Build history of the part. All positions in model axes, mm. Give positions to 0.01 mm unless a question says otherwise; leave off trailing zeros. Loops run counter-clockwise (first coordinate to the right, second up) from the corner with the lowest first, then second, coordinate; pieces in that order, holes last. Notation, with made-up numbers: (67.5, 65.25) - (75.5, 65.25) arc R24 cw to (75.5, 87.25) - close; hole circle Ø8 at (49.5, -27.5). An arc over 180 degrees is marked (long way). Return JSON: item names as keys, results as strings. Group by question number.
1) Slice it at A-A (x = -7). List the corners of the cut face in (y, z), and give its area (3 significant figures).
2) Slice it at B-B (y = -9.5). List the corners of the cut face in (x, z).
3) Drop a flat-ended pin along its axis: pin 1 (25 mm diameter, centred on x = -5.44, z = 0, fed in from -Y). Give the stop position or say it passes through.
4) Slice it at C-C (z = -1.5). List the corners of the cut face in (x, y), and give its area (3 significant figures).
5) Drill centre lines: probe 1 along Z at (x, y) = (-4.5, -39); probe 2 along Z at (x, y) = (7, -36); probe 3 along X at (y, z) = (-14.5, -2). Where is each one in solid material? Low to high. Write a range as from..to.
```python
from build123d import *

# Parameters (mm, degrees)
F1_DEPTH = 50


with BuildPart() as f1:
    # F0 (on Front) → F1 (new body)
    with BuildSketch(Plane.XZ):
        with BuildLine():
            Line((3.880708, 38.61779), (-37.671275, 38.61779))
            Line((-37.671275, 38.61779), (-37.671275, -28.584737))
            Line((-37.671275, -28.584737), (3.880708, -28.584737))
            Line((3.880708, -28.584737), (3.880708, -18.612372))
            ThreePointArc((3.880708, -18.612372), (-26.25631, 0), (3.880708, 18.612372))
            Line((3.880708, 18.612372), (3.880708, 38.61779))
        make_face()
        with BuildLine():
            Line((45.432691, 38.61779), (3.880708, 38.61779))
            Line((3.880708, 38.61779), (3.880708, 18.612372))
            ThreePointArc((3.880708, 18.612372), (12.270213, 10.937914), (15.375554, 0))
            ThreePointArc((15.375554, 0), (12.270213, -10.937914), (3.880708, -18.612372))
            Line((3.880708, -18.612372), (3.880708, -28.584737))
            Line((3.880708, -28.584737), (45.432691, -28.584737))
            Line((45.432691, -28.584737), (45.432691, 38.61779))
        make_face()
    extrude(amount=F1_DEPTH)


solid = f1.part
```
Results:
{
 "1": {"outline": "(-50, -28.58) - (0, -28.58) - (0, -20.76) - (-50, -20.76) - close; (-50, 20.76) - (0, 20.76) - (0, 38.62) - (-50, 38.62) - close", "area": "1,280 mm2"},
 "2": {"outline": "(-37.67, -28.58) - (45.43, -28.58) - (45.43, 38.62) - (-37.67, 38.62) - close; hole (3.88, -18.61) arc R20.82 ccw to (15.38, 0) arc R20.82 ccw to (3.88, 18.61) arc R20.82 ccw (long way) to start"},
 "3": {"pin 1": "through"},
 "4": {"outline": "(-37.67, -50) - (-26.2, -50) - (-26.2, 0) - (-37.67, 0) - close; (15.32, -50) - (45.43, -50) - (45.43, 0) - (15.32, 0) - close", "area": "2,080 mm2"},
 "5": {"probe 1": "-28.58..-20.79, 20.79..38.62", "probe 2": "-28.58..-16.69, 16.69..38.62", "probe 3": "-37.67..-26.16, 15.28..45.43"}
}
